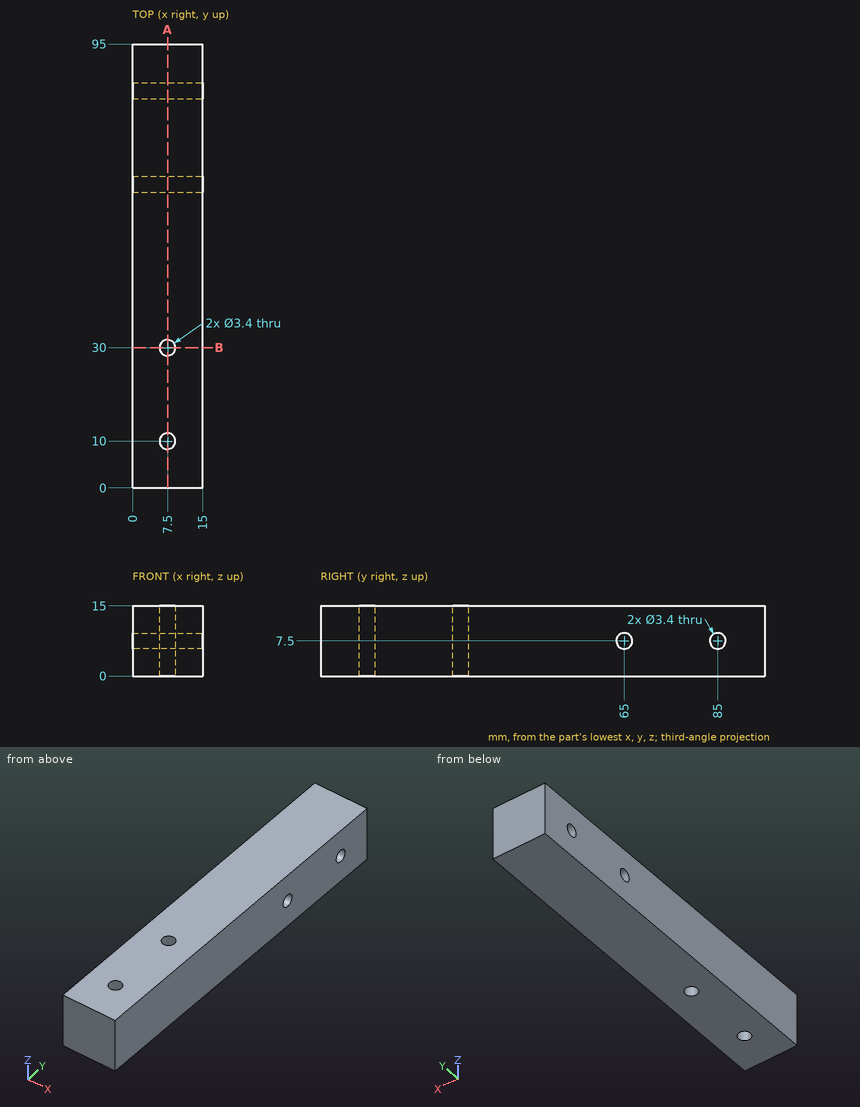
Part print with two shaded views. Sizes in mm from the minimum x, y, z corner. Coordinates: 2 decimals unless noted, no trailing zeros. Loops run counter-clockwise (first coordinate to the right, second up) from the corner with the lowest first, then second, coordinate; pieces in that order, holes last. Notation, with made-up numbers: (10, -3) - (58, -3) arc R33 cw to (58, 30) - close; hole circle Ø5 at (35.5, -5). An arc over 180 degrees is marked (long way). Write each question's results on one line, items separated by ' | '. Start each with the question number.
Q1. Slice it at A-A on x = 7.5. Give the cut face in (y, z), and give its area (3 significant figures).
Q2. Probe line 1 along Y through (x, z) = (7.25, 7.5); line 2 along Y through (x, z) = (7.25, 1); line 3 along Z through (x, y) = (7.25, 85). List the from-to ranges inside material, lowest first.
Q3. Slice it at B-B on y = 30. Give the cut face in (x, z).
Q4. Drop a flat-ended pin along its axis: pin 1 Ø2 at (x, y) = (7.5, 10) entering from +Z. Give the stop position or say it passes through.
Answer:
1) outline: (0, 0) - (8.3, 0) - (8.3, 15) - (0, 15) - close; (11.7, 0) - (28.3, 0) - (28.3, 15) - (11.7, 15) - close; (31.7, 0) - (95, 0) - (95, 15) - (31.7, 15) - close; hole circle Ø3.4 at (65, 7.5); hole circle Ø3.4 at (85, 7.5) | area: 1,300 mm2
2) line 1: y = 0 to 8.32, 11.68 to 28.32, 31.68 to 63.3, 66.7 to 83.3, 86.7 to 95 | line 2: y = 0 to 8.32, 11.68 to 28.32, 31.68 to 95 | line 3: z = 0 to 5.8, 9.2 to 15
3) outline: (0, 0) - (5.8, 0) - (5.8, 15) - (0, 15) - close; (9.2, 0) - (15, 0) - (15, 15) - (9.2, 15) - close
4) pin 1: passes through
